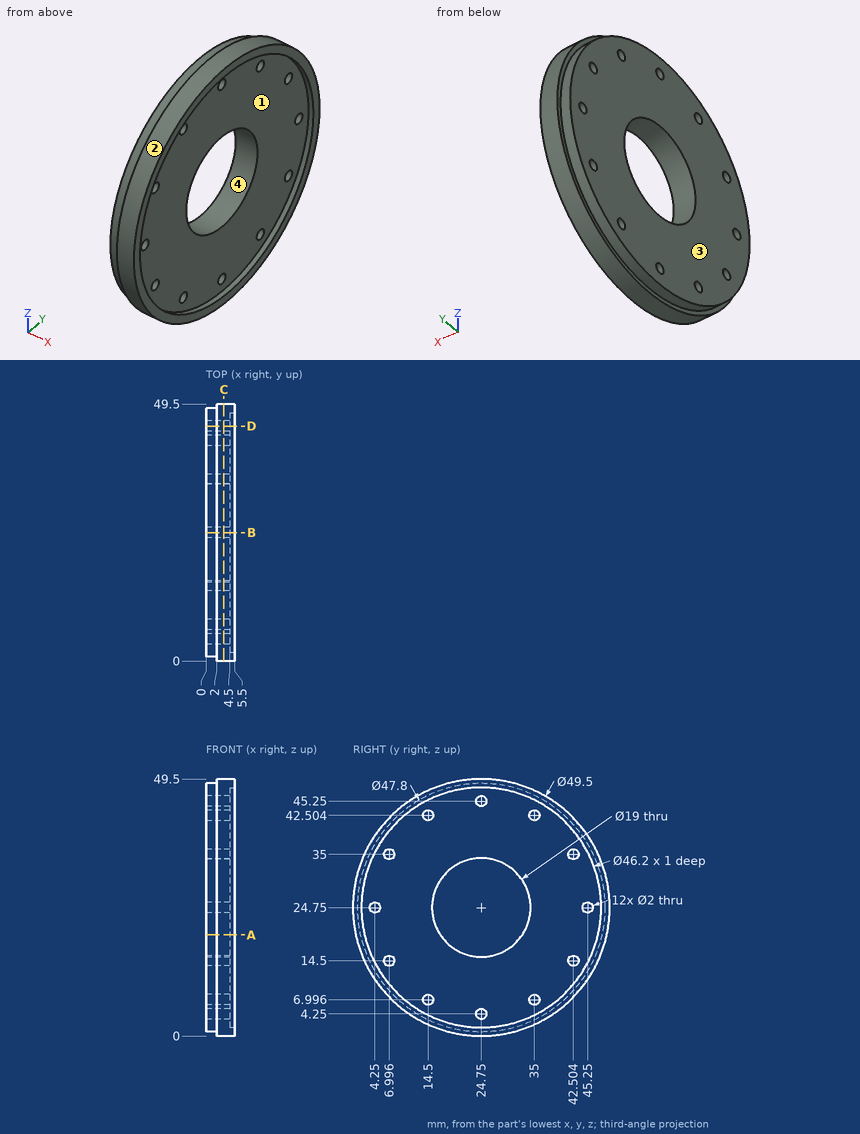
Answer from the drawing. Dimensions are ordinates in mm from the lowest x, y and z of the part. Coordinates: 2 decimals unless noted, no trailing zeros. Loops run counter-clockwise (first coordinate to the right, second up) from the corner with the lowest first, then second, coordinate; pieces in that order, holes last. Notation, with made-up numbers: (-25, 50.25) -> (21, 50.25) arc R17 cw to (21, 81.25) -> close; hole circle Ø5 at (-21.75, 61.25). An arc over 180 degrees is marked (long way). Return JSON: item names as keys, results as strings.
Item 1: For a pull along Y with two mould halves and no side action, classify the marked faces 1, 2, 3 and 4 as +Y half, -Y half, draft (parallel to the pull), parting line (faces both ways), or undercut.
Answers:
{"face 1": "undercut", "face 2": "parting line", "face 3": "draft", "face 4": "undercut"}
Item 2: Find section A-A (z = 19.5). Determine the outline of the cut face in (x, y) (1 decimal).
Answers:
{"outline": "(0, 1.4) -> (2, 1.4) -> (2, 0.6) -> (5.5, 0.6) -> (5.5, 2.3) -> (4.5, 2.3) -> (4.5, 16.8) -> (0, 16.8) -> close; (0, 32.7) -> (4.5, 32.7) -> (4.5, 47.2) -> (5.5, 47.2) -> (5.5, 48.9) -> (2, 48.9) -> (2, 48.1) -> (0, 48.1) -> close"}
Item 3: Find section D-D (y = 45.25). Determine the outline of the cut face in (x, z).
Answers:
{"outline": "(0, 12.46) -> (2, 12.46) -> (2, 10.88) -> (5.5, 10.88) -> (5.5, 14.1) -> (4.5, 14.1) -> (4.5, 23.75) -> (0, 23.75) -> close; (0, 25.75) -> (4.5, 25.75) -> (4.5, 35.4) -> (5.5, 35.4) -> (5.5, 38.62) -> (2, 38.62) -> (2, 37.04) -> (0, 37.04) -> close"}
Item 4: Find the intervals of material crossed by probe 1 along Y at (x, z) = (3.4, 35) (1 decimal); probe 2 along Y at (x, z) = (0.95, 14.5) (1 decimal), in increasing order.
Answers:
{"probe 1": "y = 2.2 to 6, 8 to 41.5, 43.5 to 47.3", "probe 2": "y = 3.2 to 6, 8 to 41.5, 43.5 to 46.3"}
Item 5: Find section B-B (y = 24.75). Determine the outline of the cut face in (x, z), plus the area to 3 significant figures.
Answers:
{"outline": "(0, 0.85) -> (2, 0.85) -> (2, 0) -> (5.5, 0) -> (5.5, 1.65) -> (4.5, 1.65) -> (4.5, 3.25) -> (0, 3.25) -> close; (0, 5.25) -> (4.5, 5.25) -> (4.5, 15.25) -> (0, 15.25) -> close; (0, 34.25) -> (4.5, 34.25) -> (4.5, 44.25) -> (0, 44.25) -> close; (0, 46.25) -> (4.5, 46.25) -> (4.5, 47.85) -> (5.5, 47.85) -> (5.5, 49.5) -> (2, 49.5) -> (2, 48.65) -> (0, 48.65) -> close", "area": "119 mm2"}
Item 6: Flat-ended cylindrical pins translate along their axes: P1, Ø1.6, axis at y = 7, z = 35, coming from the -X side; P2, Ø3, axis at y = 14.5, z = 7, coming from the -X side; P3, Ø2.5, axis at y = 4.25, z = 24.75, coming from the +X side; P4, Ø1, axis at x = 3, z = 20.5, coming from the -Y side. Find the tip coordinate at first contact, or state that the pin passes through.
Answers:
{"P1": "passes through", "P2": "stops at x = 0", "P3": "stops at x = 4.5", "P4": "stops at y = 0.29"}
Item 7: Find section C-C (x = 3.4). Count the separate pieces of the cut face and the enclosed holes in it, plus the area to 3 significant figures.
Answers:
{"separate pieces": "1", "enclosed holes": "13", "area": "1,600 mm2"}
